```python
from build123d import *

# Parameters (mm, degrees)
F2_DEPTH = 7
F3_DEPTH = 7
F4_D     = 5.5
F5_D     = 8.8


with BuildPart() as f2:
    # F1 (on Front) → F2 (new body)
    with BuildSketch(Plane.XZ):
        with BuildLine():
            ThreePointArc((-176.0360002518, 0), (-168.9649324399, 2.9289321881), (-166.0360002518, 10))
            ThreePointArc((-166.0360002518, 10), (-168.9649324399, 17.0710678119), (-176.0360002518, 20))
            ThreePointArc((-176.0360002518, 20), (-186.0360002518, 10), (-176.0360002518, 0))
        make_face()
        with BuildLine():
            Line((-264.5352196047, 20), (-240.393083981, 20))
            ThreePointArc((-240.393083981, 20), (-249.6318793158, 26.1731656999), (-247.4641517568, 37.0710678479))
            Line((-247.4641517568, 37.0710678479), (-264.5352196047, 20))
        make_face()
        with BuildLine():
            Line((-272.4173313033, -22.3205080757), (-255.0968232276, -12.3205080757))
            ThreePointArc((-255.0968232276, -12.3205080757), (-261.1688868565, -7.6612498015), (-268.757077341, -8.6602540815))
            ThreePointArc((-268.757077341, -8.6602540815), (-273.4163355396, -14.7323176668), (-272.4173313033, -22.3205080757))
        make_face()
        with BuildLine():
            Line((-255.0968232276, -12.3205080757), (-262.2100718816, 0))
            Line((-262.2100718816, 0), (-263.7570772654, 0))
            ThreePointArc((-263.7570772654, 0), (-265.0968232494, -5.0000000378), (-268.757077341, -8.6602540815))
            ThreePointArc((-268.757077341, -8.6602540815), (-261.1688868565, -7.6612498015), (-255.0968232276, -12.3205080757))
        make_face()
        with BuildLine():
            ThreePointArc((-272.4173313033, -22.3205080757), (-273.4163355396, -14.7323176668), (-268.757077341, -8.6602540815))
            ThreePointArc((-268.757077341, -8.6602540815), (-276.3452678591, -9.6592582247), (-282.4173314074, -4.9999998197))
            Line((-282.4173314074, -4.9999998197), (-272.4173313033, -22.3205080757))
        make_face()
        with BuildLine():
            ThreePointArc((-265.0968232276, 5), (-269.1126993205, 8.856057447), (-274.5681672284, 9.9670523763))
            Line((-274.5681672284, 9.9670523763), (-283.7241296417, 0.811089963))
            ThreePointArc((-283.7241296417, 0.811089963), (-283.5134253602, -2.1940081707), (-282.4173314074, -4.9999998197))
            ThreePointArc((-282.4173314074, -4.9999998197), (-276.3452678591, -9.6592582247), (-268.757077341, -8.6602540815))
            ThreePointArc((-268.757077341, -8.6602540815), (-265.0968232494, -5.0000000378), (-263.7570772654, 0))
            ThreePointArc((-263.7570772654, 0), (-264.0978190025, 2.588190451), (-265.0968232276, 5))
        make_face()
        with BuildLine():
            Line((-263.7570772654, 0), (-262.2100718816, 0))
            Line((-262.2100718816, 0), (-265.0968232276, 5))
            ThreePointArc((-265.0968232276, 5), (-264.0978190025, 2.588190451), (-263.7570772654, 0))
        make_face()
        with BuildLine():
            ThreePointArc((-176.0360002518, 0), (-186.0360002518, 10), (-176.0360002518, 20))
            Line((-176.0360002518, 20), (-240.393083981, 20))
            Line((-240.393083981, 20), (-264.5352196047, 20))
            Line((-264.5352196047, 20), (-274.5681672284, 9.9670523763))
            ThreePointArc((-274.5681672284, 9.9670523763), (-269.1126993205, 8.856057447), (-265.0968232276, 5))
            Line((-265.0968232276, 5), (-262.2100718816, 0))
            Line((-262.2100718816, 0), (-245.3697865632, 0))
            Line((-245.3697865632, 0), (-176.0360002518, 0))
        make_face()
        with BuildLine():
            Line((-283.7241296417, 0.811089963), (-274.5681672284, 9.9670523763))
            ThreePointArc((-274.5681672284, 9.9670523763), (-280.8281450773, 7.0710678119), (-283.7241296417, 0.811089963))
        make_face()
        with BuildLine():
            ThreePointArc((-282.4173314074, -4.9999998197), (-283.5134253602, -2.1940081707), (-283.7241296417, 0.811089963))
            Line((-283.7241296417, 0.811089963), (-285.0226592429, -0.4874396382))
            Line((-285.0226592429, -0.4874396382), (-282.4173314074, -4.9999998197))
        make_face()
        with BuildLine():
            Line((-274.5681672284, 9.9670523763), (-264.5352196047, 20))
            Line((-264.5352196047, 20), (-292.8194908522, 20))
            ThreePointArc((-292.8194908522, 20), (-295.7992302368, 6.1376963428), (-292.0799732137, -7.544753609))
            Line((-292.0799732137, -7.544753609), (-285.0226592429, -0.4874396382))
            Line((-285.0226592429, -0.4874396382), (-283.7241296417, 0.811089963))
            ThreePointArc((-283.7241296417, 0.811089963), (-280.8281450773, 7.0710678119), (-274.5681672284, 9.9670523763))
        make_face()
        with BuildLine():
            ThreePointArc((-292.0799732137, -7.544753609), (-283.8324896653, -17.0403017463), (-272.4173313033, -22.3205080757))
            Line((-272.4173313033, -22.3205080757), (-282.4173314074, -4.9999998197))
            Line((-282.4173314074, -4.9999998197), (-285.0226592429, -0.4874396382))
            Line((-285.0226592429, -0.4874396382), (-292.0799732137, -7.544753609))
        make_face()
        with BuildLine():
            Line((-292.8194908522, 20), (-264.5352196047, 20))
            Line((-264.5352196047, 20), (-247.4641517568, 37.0710678479))
            Line((-247.4641517568, 37.0710678479), (-204.550425378, 79.9847942268))
            ThreePointArc((-204.550425378, 79.9847942268), (-218.6925610017, 79.9847942268), (-218.6925610017, 94.1269298505))
            Line((-218.6925610017, 94.1269298505), (-236.8037936181, 76.015697234))
            Line((-236.8037936181, 76.015697234), (-251.1915228084, 61.6279680438))
            Line((-251.1915228084, 61.6279680438), (-272.8662394587, 39.9532513935))
            Line((-272.8662394587, 39.9532513935), (-287.2539686489, 25.5655222033))
            Line((-287.2539686489, 25.5655222033), (-292.8194908522, 20))
        make_face()
        with BuildLine():
            Line((-290.2788043549, 36.8543627425), (-287.2539686489, 25.5655222033))
            Line((-287.2539686489, 25.5655222033), (-272.8662394587, 39.9532513935))
            Line((-272.8662394587, 39.9532513935), (-284.1550799979, 42.9780870995))
            ThreePointArc((-284.1550799979, 42.9780870995), (-281.482408522, 41.1922651131), (-280.4491752234, 38.1484579681))
            ThreePointArc((-280.4491752234, 38.1484579681), (-284.7965442623, 33.1912336612), (-290.2788043549, 36.8543627425))
        make_face()
        with BuildLine():
            ThreePointArc((-284.1550799979, 42.9780870995), (-288.9847091293, 41.683991874), (-290.2788043549, 36.8543627425))
            ThreePointArc((-290.2788043549, 36.8543627425), (-284.7965442623, 33.1912336612), (-280.4491752234, 38.1484579681))
            ThreePointArc((-280.4491752234, 38.1484579681), (-281.482408522, 41.1922651131), (-284.1550799979, 42.9780870995))
        make_face()
        with BuildLine():
            Line((-251.1915228084, 61.6279680438), (-236.8037936181, 76.015697234))
            Line((-236.8037936181, 76.015697234), (-248.0926341574, 79.04053294))
            ThreePointArc((-248.0926341574, 79.04053294), (-245.4199626814, 77.2547109536), (-244.3867293829, 74.2109038086))
            ThreePointArc((-244.3867293829, 74.2109038086), (-248.7340984218, 69.2536795017), (-254.2163585143, 72.9168085831))
            Line((-254.2163585143, 72.9168085831), (-251.1915228084, 61.6279680438))
        make_face()
        with BuildLine():
            ThreePointArc((-244.3867293829, 74.2109038086), (-245.4199626814, 77.2547109536), (-248.0926341574, 79.04053294))
            ThreePointArc((-248.0926341574, 79.04053294), (-252.9222632888, 77.7464377145), (-254.2163585143, 72.9168085831))
            ThreePointArc((-254.2163585143, 72.9168085831), (-248.7340984218, 69.2536795017), (-244.3867293829, 74.2109038086))
        make_face()
        with BuildLine():
            ThreePointArc((-218.6925610017, 94.1269298505), (-218.6925610017, 79.9847942268), (-204.550425378, 79.9847942268))
            ThreePointArc((-204.550425378, 79.9847942268), (-202.3826978647, 83.229027715), (-201.6214931898, 87.0558620386))
            ThreePointArc((-201.6214931898, 87.0558620386), (-207.7946588662, 96.2946573637), (-218.6925610017, 94.1269298505))
        make_face()
        with BuildLine():
            ThreePointArc((-255.0968232276, -12.3205080757), (-253.2185151467, -3.8034316254), (-245.3697865632, 0))
            Line((-245.3697865632, 0), (-262.2100718816, 0))
            Line((-262.2100718816, 0), (-255.0968232276, -12.3205080757))
        make_face()
    extrude(amount=F2_DEPTH)

    # F0 (on Front) → F3 (cut, through all)
    with BuildSketch(Plane.XZ):
        with BuildLine():
            ThreePointArc((-278.0872042843, -2.5), (-272.4629820399, -4.8296291314), (-268.7570772654, 0))
            ThreePointArc((-268.7570772654, 0), (-268.927448134, 1.2940952255), (-269.4269502465, 2.5))
            ThreePointArc((-269.4269502465, 2.5), (-276.2570772654, 4.3301270189), (-278.0872042843, -2.5))
        make_face()
        with BuildLine():
            ThreePointArc((-269.4269502465, 2.5), (-268.927448134, 1.2940952255), (-268.7570772654, 0))
            ThreePointArc((-268.7570772654, 0), (-272.4629820399, -4.8296291314), (-278.0872042843, -2.5))
            Line((-278.0872042843, -2.5), (-268.0872042843, -19.8205080757))
            ThreePointArc((-268.0872042843, -19.8205080757), (-266.2570772654, -12.9903810568), (-259.4269502465, -14.8205080757))
            Line((-259.4269502465, -14.8205080757), (-269.4269502465, 2.5))
        make_face()
        with BuildLine():
            ThreePointArc((-258.7570772654, -17.3205080757), (-258.927448134, -16.0264128502), (-259.4269502465, -14.8205080757))
            ThreePointArc((-259.4269502465, -14.8205080757), (-266.2570772654, -12.9903810568), (-268.0872042843, -19.8205080757))
            ThreePointArc((-268.0872042843, -19.8205080757), (-262.4629820399, -22.1501372071), (-258.7570772654, -17.3205080757))
        make_face()
    extrude(amount=F3_DEPTH, mode=Mode.SUBTRACT)

    # F4 (through all)
    with Locations(Plane(origin=(0, 0, 0), x_dir=(1, 0, 0), z_dir=(0, 1, 0))):
        with Locations((-249.3867293829, -74.2109038086), (-285.4491752234, -38.1484579681)):
            Hole(F4_D / 2)

    # F5 (through all)
    with Locations(Plane(origin=(0, 0, 0), x_dir=(1, 0, 0), z_dir=(0, 1, 0))):
        with Locations((-176.0360002518, -10), (-211.6214931898, -87.0558620386), (-236.3702305314, -62.3071246971), (-211.0360002518, -10)):
            Hole(F5_D / 2)


solid = f2.part
```
Design review of the part built by this model. Coordinates are the model's own, in mm. A direction names the side the tool comes from. Coordinates: 2 decimals unless noted, no trailing zeros. Order: outer loops, then holes, each group sorted by start corner. A loop starts at its lowest first (then second) coordinate and runs counter-clockwise, first axis right, second up. Notation, with made-up numbers: M -36.5,13 L 12.5,13 A19 ccw 12.5,18 Z; hole C -14,-16.75 d1. An arc over 180 degrees is marked long. Answer as a JSON object with one key per item and string values. Group by question number.
1) Add section B-B, the plane y = -4.75. Write out the cut boundary in (x, z), then the cut area to 3 significant figures.
2) Tool access review of faces 1 (the cylindrical face through (-282.7, -3.55, 38.03)), 2 (the flat face through (-278.432, -3.451, 41.444)), 3 (the flat face through (-226.308, -3.451, 58.228)), 4 (the flat face through (-288.788, -3.451, 31.289)): name each direction out of +Z, -Z, +X, -X, +Y, -Y from which nothing blocks a thin tool from reaching the whole face with its end or side.
3) Add section C-C, the plane z = 49. Write out the cut boundary in (x, y), then the cut area to 3 significant figures.
4) Mouldability with a two-part tool opening along X and no side actions: class faces 5 (the flat face through (-257.292, -3.451, -13.588)), 6 (the flat face through (-290, -3.45, 22.82)), 7 (the flat face through (-273.157, -3.451, -11.039)), 8 (the flat face through (-250.5, -7, 28.8)) as pulls with the +X half, pulls with the -X half, needs draft (parallel to the pull), parting line crosses it, or undercut.
5) For pin 1 (1.5 mm diameter, centred on y = -5.5, z = 30.5, fed in from -X); pin 2 (2 mm diameter, centred on x = -243.5, y = -5, fed in from -Z); pin 3 (5.5 mm diameter, centred on x = -211.62, z = 87.06, fed in from -Y); pin 4 (2 mm diameter, centred on x = -200.5, y = -4, fed in from +Z), all flat-tipped, find the tip position at first contact; note any pin that passes through.
6) Wall thickness on L1, parallel to X at y = -0.5, z = 39; L2, parallel to X at y = -3.5, z = 88.5; L3, parallel to Z at x = -186.5, y = -3: over which ranges is each line inside the solid? List them lowest first.
7) Add section D-D, the plane x = -265. Write out the cut boundary in (y, z).
8) Add section A-A, the plane x = -179. Write out the cut boundary in (y, z), then the cut area to 3 significant figures.
Computed values:
{
 "1": {"outline": "M -292.82,20 A30 ccw -272.42,-22.32 L -268.09,-19.82 L -278.09,-2.5 A5 cw -269.43,2.5 L -259.43,-14.82 L -255.1,-12.32 A10 cw -245.37,0 L -176.04,0 A10 ccw -176.04,20 L -240.39,20 A10 cw -247.46,37.07 L -204.55,79.98 A10 ccw -218.69,94.13 L -236.8,76.02 L -248.09,79.04 A5 ccw -254.22,72.92 L -251.19,61.63 L -272.87,39.95 L -284.16,42.98 A5 ccw -290.28,36.85 L -287.25,25.57 Z; hole C -285.45,38.15 d5.5; hole C -249.39,74.21 d5.5; hole C -236.37,62.31 d8.8; hole C -211.62,87.06 d8.8; hole C -211.04,10 d8.8; hole C -176.04,10 d8.8", "area": "5,180 mm^2"},
 "2": {"face 1": "+Y, -Y", "face 2": "+Z, +Y, -Y", "face 3": "+X, +Y, -Y", "face 4": "-X, +Y, -Y"},
 "3": {"outline": "M -263.82,-7 L -235.54,-7 L -235.54,0 L -263.82,0 Z", "area": "198 mm^2"},
 "4": {"face 5": "pulls with the +X half", "face 6": "pulls with the -X half", "face 7": "undercut", "face 8": "needs draft"},
 "5": {"pin 1": "stops at x = -288.78", "pin 2": "stops at z = 0", "pin 3": "passes through", "pin 4": "stops at z = 20"},
 "6": {"L1": "x = -290.38 to -288.06, -282.83 to -245.54", "L2": "x = -224.32 to -215.78, -207.47 to -201.73", "L3": "z = 0 to 20"},
 "7": {"outline": "M -7,-5.17 L 0,-5.17 L 0,47.82 L -7,47.82 Z"},
 "8": {"outline": "M -7,0 L 0,0 L 0,6.75 L -7,6.75 Z; M -7,13.25 L 0,13.25 L 0,20 L -7,20 Z", "area": "94.5 mm^2"}
}
